Design review of the part shown in the three views and the two pictorial views. Dimensions are in mm from the part's minimum x, y and z. A direction names the side the tool comes from. Coordinates: 2 decimals unless noted, no trailing zeros. Write each loop counter-clockwise with the first axis right and the second up, starting at its lowest first coordinate (ties: lowest second). Pieces come first, ordered by that corner, then holes. Notation, with made-up numbers: M 40,-5.75 L 95,-5.75 A12 ccw 95,16.25 Z; hole C 54,21 d11. An arc over 180 degrees is marked long. Answer as a JSON object with one key per item and string values.
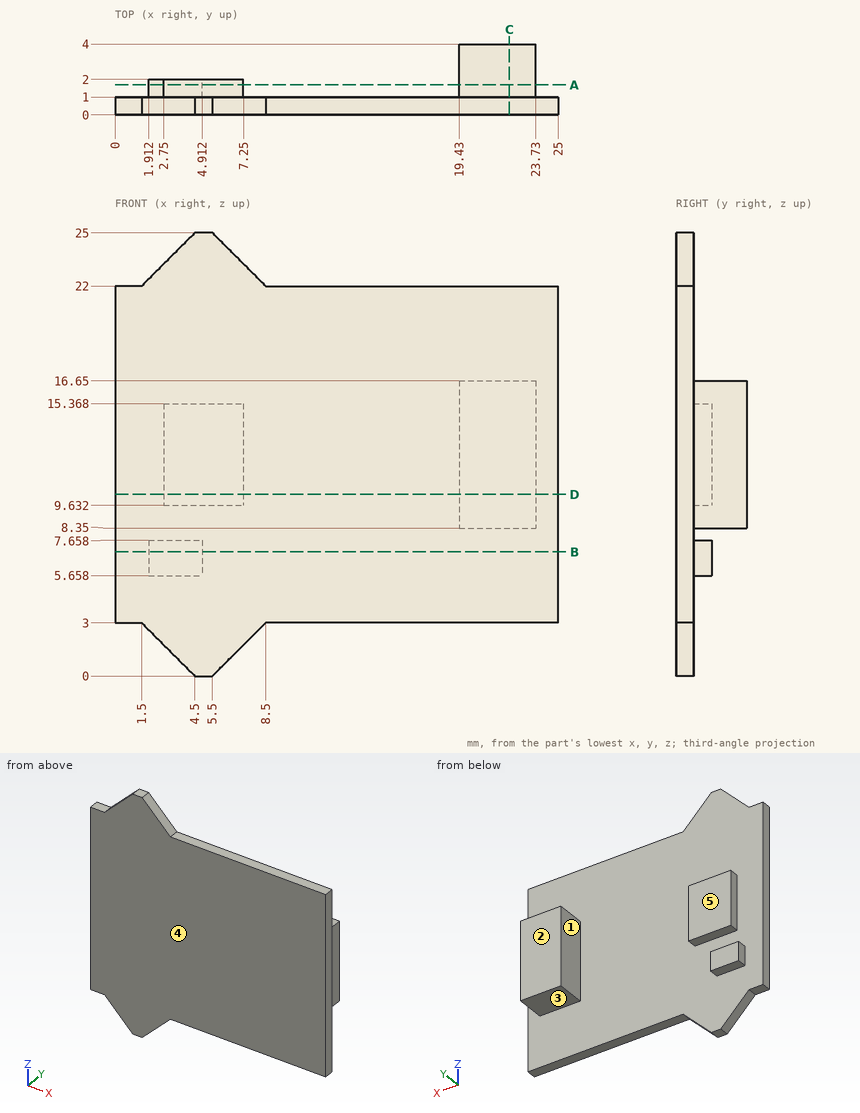
(1) Add section D-D on z = 10.25. Give the boundary of the cut face in (x, y).
Results list:
{"outline": "M 0,0 L 25,0 L 25,1 L 23.73,1 L 23.73,4 L 19.43,4 L 19.43,1 L 7.25,1 L 7.25,2 L 2.75,2 L 2.75,1 L 0,1 Z"}
(2) Add section C-C on x = 22.25. Give the boundary of the cut face in (y, z).
Results list:
{"outline": "M 0,3 L 1,3 L 1,8.35 L 4,8.35 L 4,16.65 L 1,16.65 L 1,22 L 0,22 Z"}
(3) For pin 1 Ø1.5 at (x, z) = (8.5, 8) entering from +Y; pin 2 Ø3.5 at (x, z) = (5.5, 13.5) entering from +Y; pin 3 Ø0.9 at (x, y) = (22, 3) entering from -Z, all flat-tipped, find the tip position at first contact; note any pin that passes through.
Results list:
{"pin 1": "y = 1", "pin 2": "y = 2", "pin 3": "z = 8.35"}
(4) Wall thickness on line 1 along X through (y, z) = (1.25, 14.5); line 2 along Y through (x, z) = (22.5, 18.5); line 3 along Z through (x, y) = (21, 3.25): over which ranges is each line inside the solid? List them lowest first. Write a range as from..to.
Results list:
{"line 1": "2.75..7.25, 19.43..23.73", "line 2": "0..1", "line 3": "8.35..16.65"}
(5) Add section B-B on z = 7. Give the boundary of the cut face in (x, y).
Results list:
{"outline": "M 0,0 L 25,0 L 25,1 L 4.91,1 L 4.91,2 L 1.91,2 L 1.91,1 L 0,1 Z"}
(6) Draft analysis for pull direction X (two halves, no side actions). For the marked faces 1 and 2, state which applies: released by +X, released by -X, zero draft, split by the parting line, or undercut.
Results list:
{"face 1": "undercut", "face 2": "zero draft"}
(7) For the marked faces 3, 4 and 5, list the 3-axis set-ups (+Z, -Z, +X, -X, +Y, -Y) from which the entire face can be reached by the end or side of a thin tool; tool diameter is ignored.
Results list:
{"face 3": "-Z, +X, -X, +Y", "face 4": "+Z, -Z, +X, -X, -Y", "face 5": "+Z, -Z, -X, +Y"}
(8) Add section A-A on y = 1.7. Give the boundary of the cut face in (x, z).
Results list:
{"outline": "M 1.91,5.66 L 4.91,5.66 L 4.91,7.66 L 1.91,7.66 Z; M 2.75,9.63 L 7.25,9.63 L 7.25,15.37 L 2.75,15.37 Z; M 19.43,8.35 L 23.73,8.35 L 23.73,16.65 L 19.43,16.65 Z"}
